Verification items for this drawing (mm, ordinates from the low corner). Give positions to 0.01 mm unless a question says otherwise; leave off trailing zeros. Loops run counter-clockwise (first coordinate to the right, second up) from the corner with the lowest first, then second, coordinate; pieces in that order, holes last. Notation, with made-up numbers: M 26.5,-3.5 L 59.5,-3.5 A12 cw 59.5,19.5 Z; hole C 30,46.5 d5. An arc over 180 degrees is marked long. Use a Markdown table: item, result.
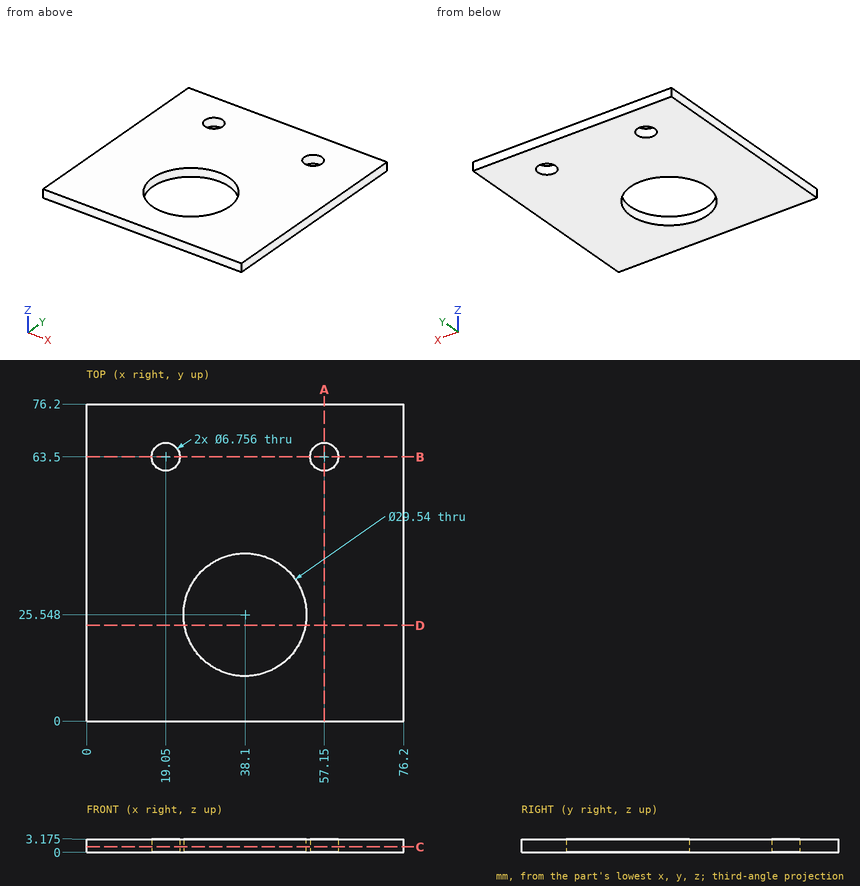
(1) Cross-section at D-D on y = 23. Record the cut outline in (x, z) (1 decimal).
Results below:
| item | result |
|---|---|
| outline | M 0,0 L 23.6,0 L 23.6,3.2 L 0,3.2 Z; M 52.6,0 L 76.2,0 L 76.2,3.2 L 52.6,3.2 Z |
(2) Cross-section at C-C on z = 1.3. Record the cut outline in (x, y).
Results below:
| item | result |
|---|---|
| outline | M 0,0 L 76.2,0 L 76.2,76.2 L 0,76.2 Z; hole C 19.05,63.5 d6.76; hole C 38.1,25.55 d29.54; hole C 57.15,63.5 d6.76 |
(3) Cross-section at B-B on y = 63.5. Record the cut outline in (x, z) (1 decimal), then the cut area to 3 significant figures.
Results below:
| item | result |
|---|---|
| outline | M 0,0 L 15.7,0 L 15.7,3.2 L 0,3.2 Z; M 22.4,0 L 53.8,0 L 53.8,3.2 L 22.4,3.2 Z; M 60.5,0 L 76.2,0 L 76.2,3.2 L 60.5,3.2 Z |
| area | 199 mm^2 |
(4) Material ranges on line 1 (Y direction, x = 19.05, z = 1.15); line 2 (Y direction, x = 38.1, z = 1.3); line 3 (X direction, y = 13.5, z = 1.5) (1 decimal), recorded low to high.
Results below:
| item | result |
|---|---|
| line 1 | 0 to 60.12, 66.88 to 76.2 |
| line 2 | 0 to 10.78, 40.32 to 76.2 |
| line 3 | 0 to 29.6, 46.6 to 76.2 |
(5) Cross-section at A-A on x = 57.15. Record the cut outline in (y, z) (1 decimal).
Results below:
| item | result |
|---|---|
| outline | M 0,0 L 60.1,0 L 60.1,3.2 L 0,3.2 Z; M 66.9,0 L 76.2,0 L 76.2,3.2 L 66.9,3.2 Z |
